Autodesk Inventor part; units mm, degrees
ref_plane "YZ Plane" through (0, 0, 0) normal (1, 0, 0) x (0, 1, 0)
ref_plane "XZ Plane" through (0, 0, 0) normal (0, 1, 0) x (-1, 0, 0)
ref_plane "XY Plane" through (0, 0, 0) normal (0, 0, 1) x (1, 0, 0)
sketch "Esboço1" plane through (0, 0, 0) normal (0, 0, 1) x (1, 0, 0)
  line L0 (-12.7424, 2.75) -> (12.7424, 2.75)
  line L1 (-12.7424, -2.75) -> (12.7424, -2.75)
  circle A0 centre (-14.9075, 0) radius 3.5
  circle A1 centre (14.9075, 0) radius 3.5
  circle A2 centre (-14.9075, 0) radius 2.5
  circle A3 centre (14.9075, 0) radius 2.5
  point P0 (0, 0)
  point P1 (0, 2.75)
  point P2 (0, -2.75)
  dimension "d7" = 7
  dimension "d5" = 2.75
  dimension "d6" = 2.75
  dimension "d9" = 14.9075
  dimension "d11" = 29.815
  dimension "d12" = 5
  dimension "d13" = 5
extrude "Extrusão1" add sketch "Esboço1" along normal mid plane 3.9 contours L0 A1 L1 A0 | A0 | A1 | A2 | A3
sketch "Esboço2" plane through (0, 0, -1.95) normal (0, 0, -1) x (-1, 0, 0)
  line L0 (-7.7154, -2.75) -> (7.7154, -2.75)
  line L1 (7.7154, -2.75) -> (7.7154, 2.75)
  line L2 (7.7154, 2.75) -> (-7.7154, 2.75)
  line L3 (-7.7154, 2.75) -> (-7.7154, -2.75)
  line L4 (-7.7154, -2.75) -> (7.7154, 2.75) construction
  line L5 (7.7154, -2.75) -> (-7.7154, 2.75) construction
  line L6 (12.7424, 2.75) -> (-12.7424, 2.75)
  line L7 (-12.7424, -2.75) -> (12.7424, -2.75)
  point P0 (0, 0)
  point P1 (0, 2.75)
  point P2 (0, -2.75)
  point P3 (7.7154, 0)
  point P4 (0, 2.75)
  dimension "d21" = 15.4307
extrude "Extrusão2" add sketch "Esboço2" along normal blind 8.04
sketch "Esboço3" plane through (0, 0, 1.95) normal (0, 0, 1) x (1, 0, 0)
  arc A0 (12.7424, -2.75) -> (12.7424, 2.75) centre (14.9075, 0) ccw
  point P0 (0, 0)
hole "Furo1" at (14.9075, 0, 1.95) direction (0, 0, -1) diameter 3.5 end through all countersink diameter 5 countersink angle 82
sketch "Esboço4" plane through (0, 0, 1.95) normal (0, 0, 1) x (1, 0, 0)
  arc A0 (-12.7424, 2.75) -> (-12.7424, -2.75) centre (-14.9075, 0) ccw
  point P0 (0, 0)
hole "Furo2" at (-14.9075, 0, 1.95) direction (0, 0, -1) diameter 3.5 end through all countersink diameter 5 countersink angle 82
sketch "Esboço5" plane through (0, 0, -9.99) normal (0, 0, -1) x (-1, 0, 0)
  arc A0 (-12.7424, 2.75) -> (-12.7424, -2.75) centre (-14.9075, 0) ccw
  circle A1 centre (-14.9075, 0) radius 3.5
  arc A2 (12.7424, -2.75) -> (12.7424, 2.75) centre (14.9075, 0) ccw
  circle A3 centre (14.9075, 0) radius 3.5
  line L0 (-12.7424, 2.75) -> (12.7424, 2.75)
  line L1 (-12.7424, -2.75) -> (12.7424, -2.75)
  circle A4 centre (-14.9075, 0) radius 2.5
  line L2 (-13.6575, -2.1651) -> (-16.1575, -2.1651)
  line L3 (-16.1575, -2.1651) -> (-17.4075, 0)
  line L4 (-17.4075, 0) -> (-16.1575, 2.1651)
  line L5 (-16.1575, 2.1651) -> (-13.6575, 2.1651)
  line L6 (-13.6575, 2.1651) -> (-12.4075, 0)
  line L7 (-12.4075, 0) -> (-13.6575, -2.1651)
  circle A5 centre (14.9075, 0) radius 2.5
  line L8 (13.6575, -2.1651) -> (12.4075, 0)
  line L9 (12.4075, 0) -> (13.6575, 2.1651)
  line L10 (13.6575, 2.1651) -> (16.1575, 2.1651)
  line L11 (16.1575, 2.1651) -> (17.4075, 0)
  line L12 (17.4075, 0) -> (16.1575, -2.1651)
  line L13 (16.1575, -2.1651) -> (13.6575, -2.1651)
  point P0 (0, 0)
  point P1 (-12.7424, -2.75)
  point P2 (-12.7424, 2.75)
  dimension "d37" = 7
extrude "Extrusão3" add sketch "Esboço5" along normal blind 3.9 contours A1 A0 | L0 A3 L1 A1 | A2 A3 | L6 A4 | A4 L7 | L5 A4 | A4 L2 | L4 A4 | A4 L3 | L11 A5 | A5 L12 | L10 A5 | A5 L13 | L9 A5 | A5 L8
properties part number "Barra1_0001_001" material "Borracha"
Can you work these out from the model? Positions are in its coordinate system, mm. A direction names the side the tool comes from. Give positions to 0.01 mm unless a question says otherwise; leave off trailing zeros. Order: outer loops, then holes, each group sorted by start corner. A loop starts at its lowest first (then second) coordinate and runs counter-clockwise, first axis right, second up. Notation, with made-up numbers: M 23.5,63 L 54.5,63 A24 cw 54.5,99 Z; hole C 9,61 d3. An arc over 180 degrees is marked long. One line per item, written item: value.
1) We'd pull the mould along Z, two halves only. Please class faces 1 (the face through (0, 0, -13.89)), 2 (the face through (-18.406, -0.11, -0.027)), 3 (the face through (7.715, 0, -6)): released by +Z, released by -Z, zero draft, split by the parting line, or undercut.
Answer sheet:
face 1: released by -Z
face 2: zero draft
face 3: undercut
2) I want a section at A-A, the plane x = -8.5. List the corners of the cut face in (y, z) for me.
Answer sheet:
outline: M -2.75,-13.89 L 2.75,-13.89 L 2.75,-9.99 L -2.75,-9.99 Z; M -2.75,-1.95 L 2.75,-1.95 L 2.75,1.95 L -2.75,1.95 Z
3) I want a section at B-B, the plane z = -12.75. List the corners of the cut face in (x, y) for me, plus the area to 3 significant figures.
Answer sheet:
outline: M -12.74,-2.75 L 12.74,-2.75 A3.5 ccw long 12.74,2.75 L -12.74,2.75 A3.5 ccw long Z; hole M -17.41,0 L -16.16,-2.17 L -13.66,-2.17 L -12.41,0 L -13.66,2.17 L -16.16,2.17 Z; hole M 12.41,0 L 13.66,-2.17 L 16.16,-2.17 L 17.41,0 L 16.16,2.17 L 13.66,2.17 Z
area: 174 mm^2
4) For P1, Ø3, axis at y = 0, z = -6.5, coming from the -X side; P2, Ø8, axis at x = 0.5, z = -3.5, coming from the -Y side, each with a flat end and sliding along its axis, tell me the tip position at first contact or that it passes through.
Answer sheet:
P1: stops at x = -7.72
P2: stops at y = -2.75
5) On a 3-axis mill with a long thin cutter (end or side, diameter ignored), from which of +Z, -Z, +X, -X, +Y, -Y can I reach the whole of each face in a straight line? I mean faces 4 (the face through (18.406, 0.11, -0.027)), 5 (the face through (-13, 0, -1.95)), 6 (the face through (-15, -2.165, -12)), 7 (the face through (0, 2.75, -6)). Say none if no direction works.
Answer sheet:
face 4: +Z, -Z
face 5: -X, +Y, -Y
face 6: -Z
face 7: +Z, -Z, +Y
6) Please list where these lines run through material, in increasing order: line 1 along X through (y, z) = (0, -0.9); line 2 along Z through (x, y) = (9.5, 0.5); line 3 along X through (y, z) = (0.75, -2.5).
Answer sheet:
line 1: x = -18.41 to -16.66, -13.16 to 13.16, 16.66 to 18.41
line 2: z = -13.89 to -9.99, -1.95 to 1.95
line 3: x = -7.72 to 7.72
7) I want a section at C-C, the plane x = -2. List the corners of the cut face in (y, z) for me.
Answer sheet:
outline: M -2.75,-13.89 L 2.75,-13.89 L 2.75,1.95 L -2.75,1.95 Z
8) I want a section at D-D, the plane z = -6. List the corners of the cut face in (x, y) for me, plus the area to 3 significant figures.
Answer sheet:
outline: M -7.72,-2.75 L 7.72,-2.75 L 7.72,2.75 L -7.72,2.75 Z
area: 84.9 mm^2
